Geometry check sheet. Reference: the model listing, model coordinates, mm. Round coordinates to 2 decimals unless told otherwise and drop trailing zeros. Order: outer loops, then holes, each group sorted by start corner. A loop starts at its lowest first (then second) coordinate and runs counter-clockwise, first axis right, second up. Notation, with made-up numbers: (-17, 10) - (-11, 10) arc R11 ccw to (-11, 30) - close; hole circle Ø10 at (34, -30). An arc over 180 degrees is marked (long way). Write each question's results on one line, items separated by ' | '.
```python
from build123d import *

# Parameters (mm, degrees)
F0_W     = 112.629154
F0_H     = 18.691752
F1_DEPTH = 31.75
F2_R     = 12.877415
F3_R     = 12.8778


with BuildPart() as f1:
    # F0 (on Front) → F1 (new body)
    with BuildSketch(Plane.XZ):
        Rectangle(F0_W, F0_H)
    extrude(amount=F1_DEPTH)

    # F2
    f2_edges = [f1.edges().sort_by_distance(p)[0] for p in [
        (56.314577, 0, 0),
        (56.314577, -31.75, 0),
    ]]
    fillet(f2_edges, radius=F2_R)

    # F3
    f3_edges = [f1.edges().sort_by_distance(p)[0] for p in [
        (-56.314577, 0, 0),
        (-56.314577, -31.75, 0),
    ]]
    fillet(f3_edges, radius=F3_R)


solid = f1.part
```
(1) Depth check by flat-ended pin: pin 1 Ø8 at (y, z) = (-8, -6) entering from -X; pin 2 Ø10 at (y, z) = (-28.5, -0.5) entering from +X; pin 3 Ø1 at (y, z) = (-28, -7) entering from +X. Enter the tip coordinate at first touch or a pass-through.
Answers follow:
pin 1: x = -56.28 | pin 2: x = 55.45 | pin 3: x = 53
(2) Section check C-C (y = -23.5). Record the cut outline in (x, z), then the cut area to 3 significant figures.
Answers follow:
outline: (-55.45, -9.35) - (55.45, -9.35) - (55.45, 9.35) - (-55.45, 9.35) - close | area: 2,070 mm²
(3) Section check B-B (x = -49). Record the cut outline in (y, z).
Answers follow:
outline: (-30.49, -9.35) - (-1.26, -9.35) - (-1.26, 9.35) - (-30.49, 9.35) - close
(4) Material ranges on line 1 (X direction, y = -25.5, z = 1); line 2 (X direction, y = -1, z = -8.5); line 3 (Y direction, x = -49, z = -5.75), recorded low to high.
Answers follow:
line 1: -54.48 to 54.48 | line 2: -48.41 to 48.41 | line 3: -30.49 to -1.26
(5) Section check A-A (z = 3). Record the cut outline in (x, y), then the cut area to 3 significant figures.
Answers follow:
outline: (-56.31, -18.87) arc R12.88 ccw to (-43.44, -31.75) - (43.44, -31.75) arc R12.88 ccw to (56.31, -18.87) - (56.31, -12.88) arc R12.88 ccw to (43.44, 0) - (-43.44, 0) arc R12.88 ccw to (-56.31, -12.88) - close | area: 3,430 mm²
